For this review, take the finished solid that the model builds, in its own axes (mm). Give positions to 0.01 mm unless a question says otherwise; leave off trailing zeros. Write each loop counter-clockwise with the first axis right and the second up, starting at its lowest first coordinate (ties: lowest second). Pieces come first, ordered by that corner, then holes. Notation, with made-up numbers: M 40.5,-23.5 L 61.5,-23.5 A11 cw 61.5,-19.5 Z; hole C -7,0 d5. An arc over 180 degrees is marked long. One line per item, written item: value. Start each with the question number.
Item 1: Consider section C-C, the plane x = 0. Write out the cut boundary in (y, z), and give its area (3 significant figures).
Item 2: Clearance check with a flat-ended pin moving along its axis: pin 1 Ø1.5 at (x, y) = (0, -28) entering from -Z. State where the tip first meets the part, or that it passes through.
Item 3: Consider section A-A, the plane z = -107. Write out the cut boundary in (x, y), and give its area (3 significant figures).
Item 4: Mouldability with a two-part tool opening along Y and no side actions: class faces 1 (the face through (0, -74, -72)), 2 (the face through (-1.5, -48, -46)), 3 (the face through (-0.021, -103.767, -14.341)), 4 (the face through (0, -40.8, -15.1)) as released by +Y, released by -Y, zero draft, split by the parting line, or undercut.
Item 5: Consider section D-D, the plane y = -13. Write out the cut boundary in (x, z).
Item 6: To check wall thickness, follow probe 1 along Z at (x, y) = (0.15, -13); probe 2 along Y at (x, z) = (0.1, -107.5); probe 3 along Z at (x, y) = (-0.8, -37). State the ranges of each line that lie inside material, in increasing order.
```python
from build123d import *

# Parameters (mm, degrees)
F0_R     = 3.5
F1_DEPTH = 1.5
F2_SIZE  = 2


with BuildPart() as f1:
    # F0 (on Right) → F1 (new body, symmetric)
    with BuildSketch(Plane.YZ):
        Polygon((-73, -73), (0, 0), (-120, 0), (-120, -26), align=None)
        with Locations((-107, -13)):
            Circle(F0_R, mode=Mode.SUBTRACT)
        with Locations((-38, -13)):
            Circle(F0_R, mode=Mode.SUBTRACT)
        Polygon((0, -120), (0, 0), (-73, -73), (-26, -120), align=None)
        with Locations((-13, -107)):
            Circle(F0_R, mode=Mode.SUBTRACT)
        with Locations((-13, -38)):
            Circle(F0_R, mode=Mode.SUBTRACT)
    extrude(amount=F1_DEPTH, both=True)

    # F2
    f2_edges = [f1.edges().sort_by_distance(p)[0] for p in [
        (0, -120, 0),
        (0, 0, 0),
        (0, 0, -120),
    ]]
    chamfer(f2_edges, length=F2_SIZE)


solid = f1.part
```
Model answer:
1. outline: M -120,-26 L -26,-120 L -2,-120 L 0,-118 L 0,-2 L -2,0 L -118,0 L -120,-2 Z; hole C -107,-13 d7; hole C -38,-13 d7; hole C -13,-107 d7; hole C -13,-38 d7
1. area: 9,820 mm2
2. pin 1: stops at z = -118.75
3. outline: M -1.5,-39 L 1.5,-39 L 1.5,-16.5 L -1.5,-16.5 Z; M -1.5,-9.5 L 1.5,-9.5 L 1.5,0 L -1.5,0 Z
3. area: 96.0 mm2
4. face 1: released by -Y
4. face 2: zero draft
4. face 3: undercut
4. face 4: undercut
5. outline: M -1.5,-120 L 1.5,-120 L 1.5,-110.5 L -1.5,-110.5 Z; M -1.5,-103.5 L 1.5,-103.5 L 1.5,-41.5 L -1.5,-41.5 Z; M -1.5,-34.5 L 1.5,-34.5 L 1.5,0 L -1.5,0 Z
6. probe 1: z = -120 to -110.5, -103.5 to -41.5, -34.5 to 0
6. probe 2: y = -38.5 to -16.46, -9.54 to 0
6. probe 3: z = -109 to -16.35, -9.65 to 0
